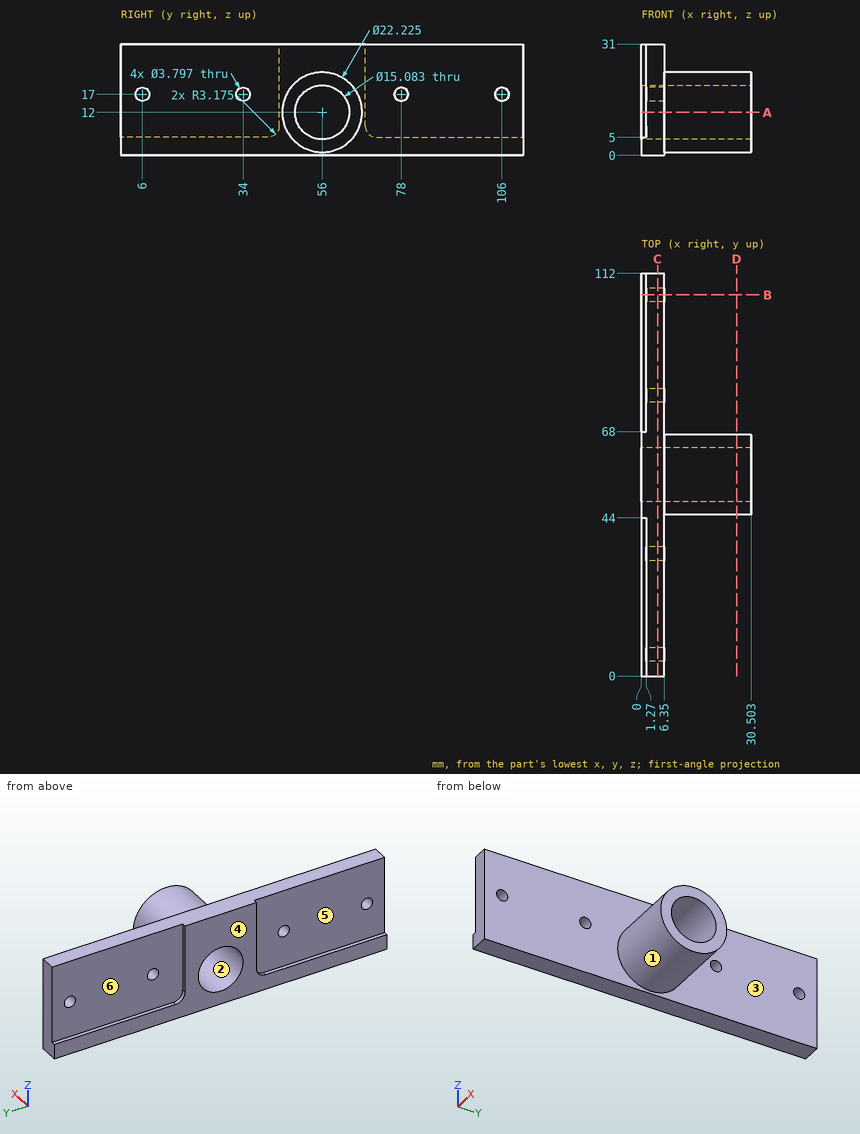
Job drawing, mm, ordinate dimensions from the low corner. One solid piece. A direction names the side the tool comes from. Give positions to 0.01 mm unless a question says otherwise; leave off trailing zeros. Write each loop counter-clockwise with the first axis right and the second up, starting at its lowest first coordinate (ties: lowest second). Pieces come first, ordered by that corner, then holes. Notation, with made-up numbers: M -18.5,60 L 4.5,60 A23 cw 4.5,79 Z; hole C 60.5,-27.5 d1. An arc over 180 degrees is marked long. Put each result on its own line as item: value. Start each with the question number.
(1) Mould opens along Y. For the marked faces 1, 2 and 3 say: +Y half, -Y half, draft (parallel to the pull), parting line (faces both ways), or undercut.
(2) Flat gauge pins, fed straight in: pin 1 Ø10 at (x, z) = (16, 5.5) entering from -Y; pin 2 Ø10 at (x, z) = (24.5, 16) entering from -Y; pin 3 Ø8 at (y, z) = (93, 19.5) entering from -X. Where does each tip first touch, or does it go through?
(3) Band-saw the part on B-B, the plane y = 106. Write the cut outline in (x, z).
(4) Probe L1, parallel to Z at x = 2.3, y = 78; L2, parallel to Z at x = 7, y = 55.5 (1 decimal); L3, parallel to Y at x = 2.4, z = 17 (1 decimal). List the from-to ranges inside material, lowest first.
(5) Band-saw the part on D-D, the plane x = 26.5. Write the cut outline in (y, z) (1 decimal).
(6) Band-saw the part on C-C, the plane x = 4.5. Write the cut outline in (y, z), and give its area (3 significant figures).
(7) Band-saw the part on A-A, the plane z = 12. Write the cut outline in (x, y), and give its area (3 significant figures).
(8) Which spindle directions (+Z, -Z, +X, -X, +Y, -Y) get a long thin tool onto all of the face, cutting with end or side? Do the marked faces 4, 5 and 6. Say none if no direction does.
Response values:
1. face 1: parting line
1. face 2: undercut
1. face 3: draft
2. pin 1: stops at y = 44.99
2. pin 2: stops at y = 44.89
2. pin 3: stops at x = 1.27
3. outline: M 0,0 L 6.35,0 L 6.35,15.1 L 1.27,15.1 L 1.27,5 L 0,5 Z; M 1.27,18.9 L 6.35,18.9 L 6.35,31 L 1.27,31 Z
4. L1: z = 0 to 15.1, 18.9 to 31
4. L2: z = 0.9 to 4.5, 19.5 to 23.1
4. L3: y = 0 to 4.1, 7.9 to 32.1, 35.9 to 50.4, 61.6 to 76.1, 79.9 to 104.1, 107.9 to 112
5. outline: C 56,12 d22.2; hole C 56,12 d15.1
6. outline: M 0,0 L 112,0 L 112,31 L 0,31 Z; hole C 6,17 d3.8; hole C 34,17 d3.8; hole C 56,12 d15.08; hole C 78,17 d3.8; hole C 106,17 d3.8
6. area: 3,250 mm2
7. outline: M 0,44 L 1.27,44 L 1.27,0 L 6.35,0 L 6.35,44.89 L 30.5,44.89 L 30.5,48.46 L 0,48.46 Z; M 0,63.54 L 30.5,63.54 L 30.5,67.11 L 6.35,67.11 L 6.35,112 L 1.27,112 L 1.27,68 L 0,68 Z
7. area: 676 mm2
8. face 4: +Z, -Z, -X, +Y, -Y
8. face 5: +Z, -X, -Y
8. face 6: +Z, -X, +Y
